The listing builds one solid part. Answer for the finished solid, in the listing's coordinates (mm). Face numbers are marked on the shaded views. A direction names the side the tool comes from. Give positions to 0.01 mm unless a question says otherwise; leave off trailing zeros. Loops run counter-clockwise (first coordinate to the right, second up) from the corner with the lowest first, then second, coordinate; pieces in that order, holes last. Notation, with made-up numbers: M -34,-31.75 L -10,-31.75 A10 cw -10,-18.75 Z; hole C 27.5,26.25 d2. An arc over 180 degrees is marked long. One line per item, written item: value. Start each with the question number.
Q1. Flat-ended cylindrical pins translate along their axes: pin 1 (3.5 mm diameter, centred on y = 2.5, z = 4.5, fed in from -X); pin 2 (3.5 mm diameter, centred on x = -7, z = 4.5, fed in from +Y); pin 3 (2.5 mm diameter, centred on x = -6, z = 4.5, fed in from -Y). Find the tip coordinate at first contact, or state that the pin passes through.
Q2. A cutting plane is placed at C-C, the plane x = -6. Determine the outline of the cut face in (y, z) (3 decimals).
Q3. For the marked faces 1, 2 and 3, determine the directions among +Z, -Z, +X, -X, +Y, -Y from which every point of the face is accessible in a straight line to the end or side of a thin tool.
Q4. A cutting plane is placed at B-B, the plane y = 0. Determine the outline of the cut face in (x, z) (3 decimals), and give its area (3 significant figures).
Q5. A cutting plane is placed at D-D, the plane z = 2.25. Determine the outline of the cut face in (x, y).
Q6. The mould has two halves that part along Y. Classify the marked faces 4, 5, 6 and 7: +Y half, -Y half, draft (parallel to the pull), parting line (faces both ways), or undercut.
Q7. Consider L1, parallel to X at y = 0, z = 5.05 (3 decimals); L2, parallel to Y at x = 0, z = 6; L3, parallel to Y at x = 1, z = 4. Determine where each line is inside the solid, lowest interval first.
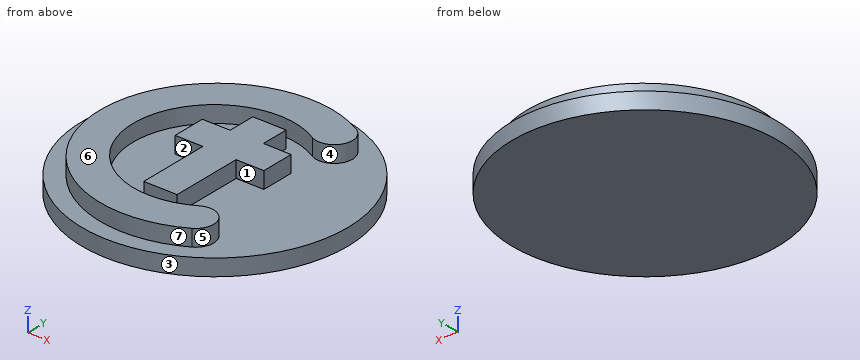
from build123d import *

# Parameters (mm, degrees)
F0_R     = 25.4
F1_DEPTH = 3.175
F2_W     = 3.175
F2_H     = 5.2916666667
F2_H_2   = 6.35
F2_W_2   = 5.2916666667
F2_H_3   = 13.7583333333
F3_DEPTH = 3.175


with BuildPart() as f1:
    # F0 (on Top) → F1 (new body)
    with BuildSketch(Plane.XY):
        Circle(F0_R)
    extrude(amount=F1_DEPTH)

    # F2 (on face) → F3 (join)
    with BuildSketch(Plane.XY.offset(3.175)):
        with BuildLine():
            ThreePointArc((7.6158286859, 13.4004975857), (12.3428438476, 14.7800857354), (10.9632556979, 19.507100897))
            ThreePointArc((10.9632556979, 19.507100897), (-21.9435583177, -0.2281861691), (11.3925767917, -19.2292929842))
            ThreePointArc((11.3925767917, -19.2292929842), (12.5870002145, -14.4702118742), (7.8279191045, -13.2757884514))
            ThreePointArc((7.8279191045, -13.2757884514), (-15.5940249542, -0.1230190166), (7.6158286859, 13.4004975857))
        make_face()
        with Locations((-1.5875, 10.0541666667)):
            Rectangle(F2_W, F2_H)
        with Locations((1.5875, 10.0541666667)):
            Rectangle(F2_W, F2_H)
        with Locations((1.5875, 4.2333333333)):
            Rectangle(F2_W, F2_H_2)
        with Locations((5.8208333333, 4.2333333333)):
            Rectangle(F2_W_2, F2_H_2)
        with Locations((-1.5875, 4.2333333333)):
            Rectangle(F2_W, F2_H_2)
        with Locations((-5.8208333333, 4.2333333333)):
            Rectangle(F2_W_2, F2_H_2)
        with Locations((-1.5875, -5.8208333333)):
            Rectangle(F2_W, F2_H_3)
        with Locations((1.5875, -5.8208333333)):
            Rectangle(F2_W, F2_H_3)
    extrude(amount=F3_DEPTH)


solid = f1.part
Answer block:
1. pin 1: x = -25.36
1. pin 2: y = 24.72
1. pin 3: y = -21.63
2. outline: M -24.681,0 L 24.681,0 L 24.681,3.175 L 21.337,3.175 L 21.337,6.35 L 14.313,6.35 L 14.313,3.175 L 7.408,3.175 L 7.408,6.35 L 1.058,6.35 L 1.058,3.175 L -14.313,3.175 L -14.313,6.35 L -21.301,6.35 L -21.301,3.175 L -24.681,3.175 Z
3. face 1: +Z, +X
3. face 2: +Z
3. face 3: +Z, -Z
4. outline: M -25.4,0 L 25.4,0 L 25.4,3.175 L 3.175,3.175 L 3.175,6.35 L -3.175,6.35 L -3.175,3.175 L -15.595,3.175 L -15.595,6.35 L -21.945,6.35 L -21.945,3.175 L -25.4,3.175 Z
4. area: 202 mm^2
5. outline: C 0,0 d50.8
6. face 4: undercut
6. face 5: undercut
6. face 6: draft
6. face 7: parting line
7. L1: -21.945 to -15.595, -3.175 to 3.175
7. L2: -22.21 to -15.47, -12.7 to 12.7, 15.47 to 22.24
7. L3: -22.2 to -15.43, -12.7 to 12.7, 15.43 to 22.23
